from build123d import *

# Parameters (mm, degrees)
EXTRUDE_1_DEPTH     = 3.2
CUT_EXTRUDE_1_DEPTH = 3.2


with BuildPart() as part:
    # Эскиз1 → Бобышка-Вытянуть1 (new body)
    with BuildSketch(Plane.XY):
        Polygon((70, -53.2), (-60, -53.2), (-80, 45), (-80, 115), (-60, 213.2), (70, 213.2), (190, 105), (190, 55), align=None)
    extrude(amount=EXTRUDE_1_DEPTH)

    # Эскиз2 → Вырез-Вытянуть1 (cut)
    with BuildSketch(Plane.XY.offset(3.2)):
        with BuildLine():
            Line((-27.5, 60), (-27.5, 100))
            ThreePointArc((-27.5, 100), (-20, 107.5), (-12.5, 100))
            Line((-12.5, 100), (-12.5, 60))
            ThreePointArc((-12.5, 60), (-20, 52.5), (-27.5, 60))
        make_face()
    extrude(amount=-CUT_EXTRUDE_1_DEPTH, mode=Mode.SUBTRACT)


solid = part.part
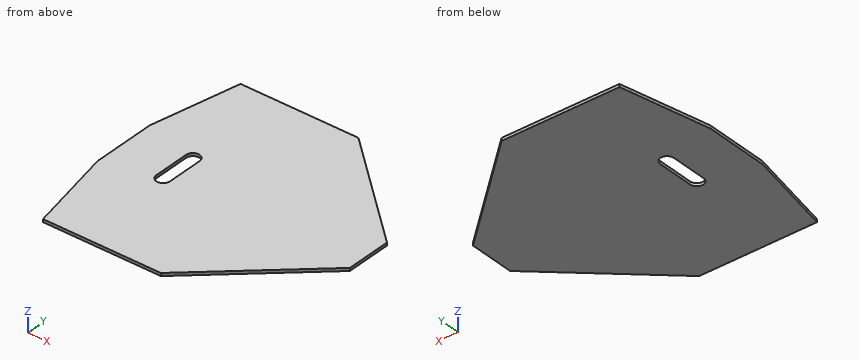
Could you check a few things on this model? Use its own coordinates, in mm. Give positions to 0.01 mm unless a question says otherwise; leave off trailing zeros. Order: outer loops, then holes, each group sorted by start corner. A loop starts at its lowest first (then second) coordinate and runs counter-clockwise, first axis right, second up. Notation, with made-up numbers: (-27.5, 35.25) - (21.5, 35.25) arc R12 ccw to (21.5, 46.25) - close; hole circle Ø1 at (66.5, -1). An arc over 180 degrees is marked (long way). Return JSON: item names as keys, results as strings. Group by question number.
Q1. Suppose I cut it at B-B, the plane x = -20. Please give me the cut outline in (y, z).
Q2. Please list where these lines run through material, in increasing order: line 1 along X through (y, z) = (76, 2.2); line 2 along X through (y, z) = (59, 3.15); line 3 along X through (y, z) = (145.5, 2.7). Write a range as [from, to].
Q3. Suppose I cut it at A-A, the plane y = 82. Please give me the cut outline in (x, z).
Q4. Suppose I cut it at D-D, the plane y = 23.5. Please give me the cut outline in (x, z).
Q5. Suppose I cut it at C-C, the plane z = 1.45. Please give me the cut outline in (x, y).
Resolved:
{
 "1": {"outline": "(-53.2, 0) - (52.5, 0) - (52.5, 3.2) - (-53.2, 3.2) - close; (107.5, 0) - (213.2, 0) - (213.2, 3.2) - (107.5, 3.2) - close"},
 "2": {"line 1": "x = [-80, -27.5], [-12.5, 190]", "line 2": "x = [-80, -27.43], [-12.57, 190]", "line 3": "x = [-73.79, 145.08]"},
 "3": {"outline": "(-80, 0) - (-27.5, 0) - (-27.5, 3.2) - (-80, 3.2) - close; (-12.5, 0) - (190, 0) - (190, 3.2) - (-12.5, 3.2) - close"},
 "4": {"outline": "(-75.62, 0) - (155.06, 0) - (155.06, 3.2) - (-75.62, 3.2) - close"},
 "5": {"outline": "(-80, 45) - (-60, -53.2) - (70, -53.2) - (190, 55) - (190, 105) - (70, 213.2) - (-60, 213.2) - (-80, 115) - close; hole (-27.5, 60) arc R7.5 ccw to (-12.5, 60) - (-12.5, 100) arc R7.5 ccw to (-27.5, 100) - close"}
}
